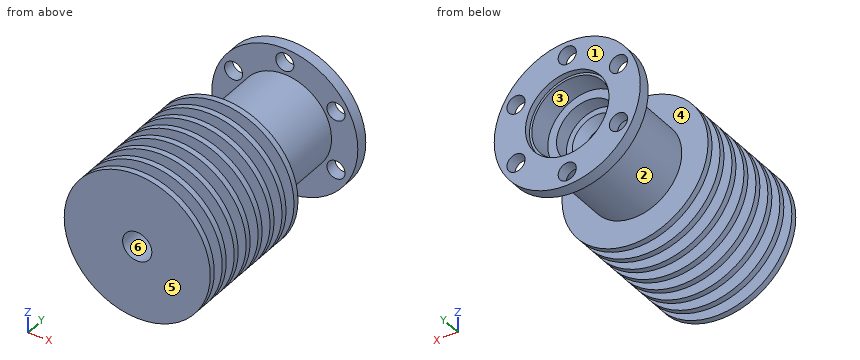
from build123d import *

# Parameters (mm, degrees)
SALIENTE_EXTRUIR1_START = -1
CROQUIS3_R              = 12.5
CROQUIS3_R_2            = 3.25
SALIENTE_EXTRUIR1_DEPTH = 1
MATRIZL1_COUNT          = 8
MATRIZL1_PITCH          = 3
CORTAR_EXTRUIR1_REACH   = 44.819
CROQUIS5_R              = 1.55
MATRIZC1_COUNT          = 6
CHAFL_N3_SIZE           = 0.3
CHAFL_N3_SIZE2          = 0.519615242
CROQUIS6_R              = 7.15
CORTAR_EXTRUIR2_DEPTH   = 1
CHAFL_N2_SIZE           = 0.15
CHAFL_N2_SIZE2          = 0.259807621
CHAFL_N4_SIZE           = 1
CHAFL_N4_SIZE2          = 1.732050808


with BuildPart() as part:
    # Croquis1 → Revolución1 (revolve)
    with BuildSketch(Plane.XY, mode=Mode.PRIVATE) as revoluci_n1_sk:
        Polygon((0, 0), (6, 0), (6, 9), (5.25, 9), (5.25, 12), (4.75, 12), (4.75, 22), (8, 22), (8, 37), (12.5, 37), (12.5, 39), (0, 39), align=None)
    revolve(revoluci_n1_sk.sketch.rotate(Axis((0, 39, 0), (0, -1, 0)), 90), axis=Axis((0, 39, 0), (0, -1, 0)))

    # Croquis2 → Cortar-Revolución1 (revolve, cut)
    with BuildSketch(Plane.XY, mode=Mode.PRIVATE) as cortar_revoluci_n1_sk:
        Polygon((0, 0), (2.5, 0), (2.5, 9), (1.7, 9), (1.7, 11), (3.25, 11), (3.25, 31.5), (5.25, 31.5), (5.25, 34), (6.75, 34), (6.75, 39), (0, 39), align=None)
    revolve(cortar_revoluci_n1_sk.sketch.rotate(Axis((0, 0, 0), (0, 1, 0)), 90), axis=Axis((0, 0, 0), (0, 1, 0)), mode=Mode.SUBTRACT)

    # Croquis3 → Saliente-Extruir1 (add)
    with BuildSketch(Plane.XZ.offset(SALIENTE_EXTRUIR1_START)):
        with Locations(Location((0, 0, 0), (0, 0, 90))):
            Circle(CROQUIS3_R)
        with Locations(Location((0, 0, 0), (0, 0, 270))):
            Circle(CROQUIS3_R_2, mode=Mode.SUBTRACT)
    saliente_extruir1 = extrude(amount=SALIENTE_EXTRUIR1_DEPTH)

    # MatrizL1: Saliente-Extruir1 ×8
    with Locations(*[(0, i * MATRIZL1_PITCH, 0) for i in range(1, MATRIZL1_COUNT)]):
        add(saliente_extruir1)

    # Croquis5 → Cortar-Extruir1 (cut, up to next)
    with BuildSketch(Plane(origin=(0, 39, 0), x_dir=(1, 0, 0), z_dir=(0, 1, 0)), mode=Mode.PRIVATE) as cortar_extruir1_sk1:
        with Locations(Location((0, 10.125, 0), (0, 0, 180))):
            Circle(CROQUIS5_R)
    cortar_extruir1_tool1 = extrude(cortar_extruir1_sk1.sketch, amount=-CORTAR_EXTRUIR1_REACH, mode=Mode.PRIVATE) & part.part
    cortar_extruir1 = cortar_extruir1_tool1.solids().sort_by_distance((0, 39, -10.125))[0]
    add(cortar_extruir1, mode=Mode.SUBTRACT)

    # MatrizC1: Cortar-Extruir1 ×6 about axis
    matrizc1_axis = Axis((0, 0, 0), (0, 1, 0))
    for i in range(1, MATRIZC1_COUNT):
        add(cortar_extruir1.rotate(matrizc1_axis, i * 360 / MATRIZC1_COUNT), mode=Mode.SUBTRACT)

    # Chaflán3
    chafl_n3_edges = [part.edges().sort_by_distance(p)[0] for p in [
        (0, 11, 1.7),
    ]]
    chafl_n3_side = [part.faces().sort_by_distance(p)[0] for p in [
        (0, 11, 1.791923882),
    ]]
    chamfer(chafl_n3_edges, length=CHAFL_N3_SIZE, length2=CHAFL_N3_SIZE2, reference=chafl_n3_side[0])

    # Croquis6 → Cortar-Extruir2 (cut)
    with BuildSketch(Plane(origin=(0, 39, 0), x_dir=(1, 0, 0), z_dir=(0, 1, 0))):
        with Locations(Location((0, 0, 0), (0, 0, 180))):
            Circle(CROQUIS6_R)
    extrude(amount=-CORTAR_EXTRUIR2_DEPTH, mode=Mode.SUBTRACT)

    # Chaflán2
    chafl_n2_edges = [part.edges().sort_by_distance(p)[0] for p in [
        (0, 9, 1.7),
    ]]
    chafl_n2_side = [part.faces().sort_by_distance(p)[0] for p in [
        (0, 9, 2.429289322),
    ]]
    chamfer(chafl_n2_edges, length=CHAFL_N2_SIZE, length2=CHAFL_N2_SIZE2, reference=chafl_n2_side[0])

    # Chaflán4
    chafl_n4_edges = [part.edges().sort_by_distance(p)[0] for p in [
        (0, 31.5, 3.25),
    ]]
    chafl_n4_side = [part.faces().sort_by_distance(p)[0] for p in [
        (0, 31.5, 3.398492424),
    ]]
    chamfer(chafl_n4_edges, length=CHAFL_N4_SIZE, length2=CHAFL_N4_SIZE2, reference=chafl_n4_side[0])


solid = part.part
The listing builds one solid part. Answer for the finished solid, in the listing's coordinates (mm). Face numbers are marked on the shaded views. A direction names the side the tool comes from. Round coordinates to 2 decimals unless told otherwise and drop trailing zeros. Loops run counter-clockwise (first coordinate to the right, second up) from the corner with the lowest first, then second, coordinate; pieces in that order, holes last. Notation, with made-up numbers: M 44,50 L 83,50 A35 cw 83,82 Z; hole C 33.25,57 d2. An arc over 180 degrees is marked long. Return JSON: item names as keys, results as strings.
Q1. Find section A-A, the plane y = 3.5. Determine the outline of the cut face in (x, z).
Results list:
{"outline": "C 0,0 d25; hole C 0,0 d5"}
Q2. The mould has two halves that part along Z. Classify the marked faces 1, 2 and 3: released by +Z, released by -Z, zero draft, split by the parting line, or undercut.
Results list:
{"face 1": "zero draft", "face 2": "split by the parting line", "face 3": "undercut"}
Q3. Find the intervals of material crossed by line 1 along Y through (x, z) = (-5.25, -1.75); line 2 along Z through (x, y) = (-0.25, 12.5); line 3 along X through (y, z) = (15.25, 0), in increasing order. Write a range as from..to.
Results list:
{"line 1": "y = 0..10, 12..13, 15..16, 18..19, 21..34", "line 2": "z = -12.5..-3.24, 3.24..12.5", "line 3": "x = -12.5..-3.25, 3.25..12.5"}
Q4. Which of the six approach directions +Z, -Z, +X, -X, +Y, -Y give full straight-line access (tool end or side, diameter ignored) to the marked faces 4, 5 and 6?
Results list:
{"face 4": "none", "face 5": "+Z, -Z, +X, -X, -Y", "face 6": "-Y"}
Q5. Find section B-B, the plane x = 0. State how many separate pieces and enclosed holes the cut face has, plus the area to 3 significant figures.
Results list:
{"separate pieces": "4", "enclosed holes": "0", "area": "346 mm2"}
Q6. Each of these flat-tipped pins is pushed along its axis until it touches: pin 1 Ø2 at (x, y) = (5, 27.5) entering from -Z; pin 2 Ø4 at (x, y) = (8.5, 12) entering from -Z; pin 3 Ø8 at (y, z) = (18, -9.5) entering from -X (3 decimals); pin 4 Ø2 at (x, z) = (0, 0) entering from -Y. Where does it stop, or does it pass through?
Results list:
{"pin 1": "stops at z = -6.93", "pin 2": "stops at z = -10.68", "pin 3": "stops at x = -11.225", "pin 4": "passes through"}
Q7. Find section C-C, the plane y = 29. Determine the outline of the cut face in (x, z).
Results list:
{"outline": "C 0,0 d16; hole C 0,0 d6.5"}
